from build123d import *

# Parameters (mm, degrees)
EXTRUDE_1_DEPTH          = 6
SKETCH_2_R               = 3
CUT_EXTRUDE_1_DEPTH      = 7
EXTRUDE_START            = -3.991967
EXTRUDE_2_DEPTH          = 3.991967
PATTERN_CIRCULAR_1_COUNT = 2


with BuildPart() as part:
    # Sketch 1 → Extrude 1 (new body)
    with BuildSketch(Plane.XY):
        with BuildLine():
            Line((-4.5, 0), (-4.5, -18.2))
            Line((-4.5, -18.2), (-3, -18.2))
            Line((-3, -18.2), (-3, -14.6))
            ThreePointArc((-3, -14.6), (-1.968245837, -12.85), (-3, -11.1))
            Line((-3, -11.1), (-3, -10))
            Line((-3, -10), (3, -10))
            Line((3, -10), (3, -11.1))
            ThreePointArc((3, -11.1), (1.968245837, -12.85), (3, -14.6))
            Line((3, -14.6), (3, -18.2))
            Line((3, -18.2), (4.5, -18.2))
            Line((4.5, -18.2), (4.5, 0))
            ThreePointArc((4.5, 0), (0, 4.5), (-4.5, 0))
        make_face()
    extrude_1 = extrude(amount=EXTRUDE_1_DEPTH)

    # Sketch 2 → Cut-Extrude 1 (cut, through all)
    with BuildSketch(Plane.XY):
        Circle(SKETCH_2_R)
        with BuildLine():
            Line((-3, -8.75), (-3, -3.354101966))
            ThreePointArc((-3, -3.354101966), (0, -4.5), (3, -3.354101966))
            Line((3, -3.354101966), (3, -8.75))
            Line((3, -8.75), (-3, -8.75))
        make_face()
    cut_extrude_1 = extrude(amount=CUT_EXTRUDE_1_DEPTH, mode=Mode.SUBTRACT)

    # Sketch 3 → Extrude 2 (add)
    with BuildSketch(Plane.XZ.offset(18.2).offset(EXTRUDE_START)):
        with BuildLine():
            Line((-3, 6), (-3, 0))
            Line((-3, 0), (-2.5, 1))
            Line((-2.5, 1), (-2.5, 1.5))
            ThreePointArc((-2.5, 1.5), (-2.757359313, 3), (-2.5, 4.5))
            Line((-2.5, 4.5), (-2.5, 5))
            Line((-2.5, 5), (-3, 6))
        make_face()
        with BuildLine():
            Line((3, 0), (2.5, 1))
            Line((2.5, 1), (2.5, 1.5))
            ThreePointArc((2.5, 1.5), (2.757359313, 3), (2.5, 4.5))
            Line((2.5, 4.5), (2.5, 5))
            Line((2.5, 5), (3, 6))
            Line((3, 6), (3, 0))
        make_face()
    extrude_2 = extrude(amount=EXTRUDE_2_DEPTH)

    # Pattern Circular 1: Extrude 1, Cut-Extrude 1, Extrude 2 ×2 about axis
    pattern_circular_1_axis = Axis((0, 0, 0), (0, 0, 1))
    for i in range(1, PATTERN_CIRCULAR_1_COUNT):
        add(extrude_1.rotate(pattern_circular_1_axis, i * 360 / PATTERN_CIRCULAR_1_COUNT))
        add(cut_extrude_1.rotate(pattern_circular_1_axis, i * 360 / PATTERN_CIRCULAR_1_COUNT), mode=Mode.SUBTRACT)
        add(extrude_2.rotate(pattern_circular_1_axis, i * 360 / PATTERN_CIRCULAR_1_COUNT))


solid = part.part
The listing builds one solid part. Answer for the finished solid, in the listing's coordinates (mm). A direction names the side the tool comes from. Give positions to 0.01 mm unless a question says otherwise; leave off trailing zeros. Loops run counter-clockwise (first coordinate to the right, second up) from the corner with the lowest first, then second, coordinate; pieces in that order, holes last. Notation, with made-up numbers: M 72.5,78 L 89.5,78 A15 cw 89.5,89 Z; hole C 81,82.5 d11. An arc over 180 degrees is marked long. Answer as CSV lines item,"result".
Item 1: The mould has two halves that part along Y. Classify faces 1 (the flat face through (-4.5, 0, 3)), 2 (the flat face through (-3, -10.6, 3)), 3 (the flat face through (3, -10.5, 3)), 4 (the flat face through (4, 18.2, 3)): released by +Y, released by -Y, zero draft, split by the parting line, or undercut.
Values follow:
face 1,"zero draft"
face 2,"undercut"
face 3,"undercut"
face 4,"released by +Y"
Item 2: The part is cut by section C-C (y = -15). Give the vertices of the cut face in (x, z).
Values follow:
outline,"M -4.5,0 L -3,0 L -2.5,1 L -2.5,1.5 A4.5 cw -2.5,4.5 L -2.5,5 L -3,6 L -4.5,6 Z; M 2.5,1 L 3,0 L 4.5,0 L 4.5,6 L 3,6 L 2.5,5 L 2.5,4.5 A4.5 cw 2.5,1.5 Z"
Item 3: Which of the six approach directions +Z, -Z, +X, -X, +Y, -Y give full straight-line access (tool end or side, diameter ignored) to faces 5 (the flat face through (4, 0, 6)), 6 (the flat face through (-3, -6, 3)), 7 (the cylindrical face through (2.757, 16.176, 2.979)), 8 (the flat face through (2.753, 16.176, 0.493)), 9 (the flat face through (-2.746, -16.176, 5.493))?
Values follow:
face 5,"+Z, +X, -X, +Y, -Y"
face 6,"+Z, -Z"
face 7,"+Y"
face 8,"-Z, +Y"
face 9,"+Z, -Y"
Item 4: The part is cut by section A-A (y = 0). Give the vertices of the cut face in (x, z).
Values follow:
outline,"M -4.5,0 L -3,0 L -3,6 L -4.5,6 Z; M 3,0 L 4.5,0 L 4.5,6 L 3,6 Z"
Item 5: The part is cut by section B-B (x = 0). Give the vertices of the cut face in (y, z).
Values follow:
outline,"M -10,0 L -8.75,0 L -8.75,6 L -10,6 Z; M -4.5,0 L -3,0 L -3,6 L -4.5,6 Z; M 3,0 L 4.5,0 L 4.5,6 L 3,6 Z; M 8.75,0 L 10,0 L 10,6 L 8.75,6 Z"
Item 6: Given pin 1 Ø3 at (x, z) = (1, 2.5) entering from +Y; pin 2 Ø1.8 at (x, z) = (0, 2.5) entering from +Y; pin 3 Ø1 at (x, z) = (1, 1) entering from -Y, each flat-ended and moving along its own axis, determine where each tip first touches the part or whether it passes through.
Values follow:
pin 1,"stops at y = 14.21"
pin 2,"stops at y = 10"
pin 3,"stops at y = -10"
Item 7: Straight lines are drawn through the part: line 1 along Y through (x, z) = (0, 3.35); line 2 along X through (y, z) = (7.5, 2.5); line 3 along Y through (x, z) = (-0.75, 2.25). For each, find the intervals that lie inside material, in ascending order. Write a range as [from, to].
Values follow:
line 1,"y = [-10, -8.75], [-4.5, -3], [3, 4.5], [8.75, 10]"
line 2,"x = [-4.5, -3], [3, 4.5]"
line 3,"y = [-10, -8.75], [-4.44, -2.9], [2.9, 4.44], [8.75, 10]"
